```python
from build123d import *

# Parameters (mm, degrees)
F6_R      = 4.5
F6_R_2    = 3.5
F9_DEPTH  = 4
F0_R      = 8
F0_R_2    = 6
F10_DEPTH = 3
F2_R      = 8
F4_R      = 4.5


with BuildPart() as f8:
    # F7 (on Front) → F8 (revolve)
    with BuildSketch(Plane.XZ):
        with BuildLine():
            Line((4.5, 23), (3, 23))
            add(Edge.make_bspline(
                [(3, 23), (3.5, 21.6666666667), (4.5, 19), (3.5, 16.3333333333), (3, 15)],
                knots=[0, 0, 0, 0, 0.5, 1, 1, 1, 1], degree=3))
            Line((3, 15), (4.5, 15))
            add(Edge.make_bspline(
                [(4.5, 23), (5, 21.6666666667), (6, 19), (5, 16.3333333333), (4.5, 15)],
                knots=[0, 0, 0, 0, 0.5, 1, 1, 1, 1], degree=3))
        make_face()
    revolve(axis=Axis((0, 0, 19), (0, 0, 1)))

    # F6 (on offset) → F9 (join, through all)
    with BuildSketch(Plane.XY.offset(15)):
        Circle(F6_R)
        Circle(F6_R_2, mode=Mode.SUBTRACT)
    extrude(amount=-F9_DEPTH)



with BuildPart() as f10:
    # F0 (on Top) → F10 (new body, through all)
    with BuildSketch(Plane.XY):
        Circle(F0_R)
        Circle(F0_R_2, mode=Mode.SUBTRACT)
    extrude(amount=F10_DEPTH)


with BuildPart() as f8_1:
    add(f8.part)

    add(f10.part)  # F11 merges F10
    # F2 (on offset) → F11 section 0
    with BuildSketch(Plane.XY.offset(3)):
        Circle(F2_R)
    # F4 (on offset) → F11 section 1
    with BuildSketch(Plane.XY.offset(11)):
        Circle(F4_R)
    loft()


solid = f8_1.part
```
Input: part model. Units: mm. Frame: model coordinates. A direction names the side the tool comes from. Give positions to 0.01 mm unless a question says otherwise; leave off trailing zeros. Loops run counter-clockwise (first coordinate to the right, second up) from the corner with the lowest first, then second, coordinate; pieces in that order, holes last. Notation, with made-up numbers: M 55.25,30.5 L 95.25,30.5 A26 ccw 95.25,55.5 Z; hole C 24,83.5 d6. An arc over 180 degrees is marked long. Answer as CSV lines item,"result". Start each with the question number.
1. Pin query (flat end, axial travel): P1, Ø4, axis at y = 4, z = 6.5, coming from the -X side; P2, Ø1.5, axis at y = -5.5, z = 19.5, coming from the +X side; P3, Ø3, axis at x = -1.5, y = 2.5, coming from the -Z side. Return the tip coordinate at first contact, or that it passes through.
2. Reachability of faces 4 (the face through (-6, 0, 1)), 5 (the face through (-0.59, 4.46, 13.03)), 6 (the face through (1, -3, 23)) from +Z, -Z, +X, -X, +Y, -Y: full face, straight path, thin tool, end or side. Return the list, or none.
3. Line query: L1, parallel to Z at x = 2.5, y = -0.25; L2, parallel to Y at x = 0.75, z = 11.75; L3, parallel to X at y = -1.75, z = 12. Output: solid intervals per line, ascending.
4. Section A-A on z = 13.25. Return loops of the section in (x, y), plus the area to 3 significant figures.
5. Pull-direction query (Y, two-part tool) for faces 1 (the face through (-2, 6, 0)), 2 (the face through (0, 0, 3)), 3 (the face through (-1.73, -7.81, 1.48)); classes: released by +Y, released by -Y, zero draft, split by the parting line, or undercut.
Computed values:
1,P1,"stops at x = -6.6"
1,P2,"stops at x = 2.73"
1,P3,"stops at z = 3"
2,face 4,"-Z"
2,face 5,"none"
2,face 6,"+Z, +X, -X, +Y, -Y"
3,L1,"z = 3 to 11"
3,L2,"y = -4.44 to -3.42, 3.42 to 4.44"
3,L3,"x = -4.15 to -3.03, 3.03 to 4.15"
4,outline,"C 0,0 d9; hole C 0,0 d7"
4,area,"25.1 mm²"
5,face 1,"zero draft"
5,face 2,"undercut"
5,face 3,"split by the parting line"
